The model under review builds one solid part; all positions refer to its coordinate system, in mm. Coordinates: 2 decimals unless noted, no trailing zeros. Order: outer loops, then holes, each group sorted by start corner. A loop starts at its lowest first (then second) coordinate and runs counter-clockwise, first axis right, second up. Notation, with made-up numbers: (69.25, 87.5) - (73.25, 87.5) arc R24 ccw to (73.25, 123.5) - close; hole circle Ø6 at (53, 33.25). An arc over 180 degrees is marked (long way). Answer in a Markdown table with one row per item.
```python
from build123d import *

# Parameters (mm, degrees)
ESQUISSE1_W                  = 70
ESQUISSE1_H                  = 118
BOSS_EXTRU_1_DEPTH           = 3
BOSS_EXTRU_2_DEPTH           = 3
CONG_1_R                     = 3
CONG_2_R                     = 3
CONG_3_R                     = 5
ESQUISSE3_W                  = 70
ESQUISSE3_H                  = 118
BOSS_EXTRU_3_DEPTH           = 3
CONG_4_R                     = 3
ENL_V_MAT_EXTRU_1_DEPTH      = 197.603662224
ENL_V_MAT_EXTRU_1_DEPTH_BACK = 197.603662224


with BuildPart() as part:
    # Esquisse1 → Boss.-Extru.1 (new body)
    with BuildSketch(Plane.XY):
        with Locations((35, 59)):
            Rectangle(ESQUISSE1_W, ESQUISSE1_H)
    extrude(amount=BOSS_EXTRU_1_DEPTH)

    # Esquisse2 → Boss.-Extru.2 (add)
    with BuildSketch(Plane.XY.offset(3)):
        Polygon((0, 118), (7.279404685, 138), (62.720595315, 138), (70, 118), align=None)
        Polygon((0, 118), (-12.5, 113.450372072), (-12.5, 4.549627928), (0, 0), align=None)
        Polygon((65.450372072, -12.5), (4.549627928, -12.5), (0, 0), (70, 0), align=None)
    extrude(amount=-BOSS_EXTRU_2_DEPTH)

    # Congé1
    cong_1_edges = [part.edges().sort_by_distance(p)[0] for p in [
        (-12.5, 4.549627928, 1.5),
        (-12.5, 113.450372072, 1.5),
    ]]
    fillet(cong_1_edges, radius=CONG_1_R)

    # Congé2
    cong_2_edges = [part.edges().sort_by_distance(p)[0] for p in [
        (65.450372072, -12.5, 1.5),
        (4.549627928, -12.5, 1.5),
    ]]
    fillet(cong_2_edges, radius=CONG_2_R)

    # Congé3
    cong_3_edges = [part.edges().sort_by_distance(p)[0] for p in [
        (7.279404685, 138, 1.5),
        (62.720595315, 138, 1.5),
    ]]
    fillet(cong_3_edges, radius=CONG_3_R)

    # Esquisse3 → Boss.-Extru.3 (add)
    with BuildSketch(Plane.XY.offset(3)):
        with Locations((105, 59)):
            Rectangle(ESQUISSE3_W, ESQUISSE3_H)
    extrude(amount=-BOSS_EXTRU_3_DEPTH)

    # Congé4
    cong_4_edges = [part.edges().sort_by_distance(p)[0] for p in [
        (140, 118, 1.5),
        (140, 0, 1.5),
    ]]
    fillet(cong_4_edges, radius=CONG_4_R)

    # Esquisse4 → Enlèv. mat.-Extru.1 (cut, two sides: drawn at the far end of the back side and taken through both)
    with BuildSketch(Plane.XY.offset(3).offset(-ENL_V_MAT_EXTRU_1_DEPTH_BACK)):
        with BuildLine():
            Line((80, 60), (130, 60))
            ThreePointArc((130, 60), (131, 59), (130, 58))
            Line((130, 58), (80, 58))
            ThreePointArc((80, 58), (79, 59), (80, 60))
        make_face()
        with BuildLine():
            Line((80, 40), (130, 40))
            ThreePointArc((130, 40), (131, 39), (130, 38))
            Line((130, 38), (80, 38))
            ThreePointArc((80, 38), (79, 39), (80, 40))
        make_face()
        with BuildLine():
            Line((80, 20), (130, 20))
            ThreePointArc((130, 20), (131, 19), (130, 18))
            Line((130, 18), (80, 18))
            ThreePointArc((80, 18), (79, 19), (80, 20))
        make_face()
    extrude(amount=ENL_V_MAT_EXTRU_1_DEPTH + ENL_V_MAT_EXTRU_1_DEPTH_BACK, mode=Mode.SUBTRACT)


solid = part.part
```
Item 1: We need section B-B, the plane x = 76.5. Write out the cut boundary in (y, z), then the cut area to 3 significant figures.
Check values:
| item | result |
|---|---|
| outline | (0, 0) - (118, 0) - (118, 3) - (0, 3) - close |
| area | 354 mm^2 |
Item 2: We need section A-A, the plane z = 0.6. State how many separate pieces and enclosed holes the cut face has, then the cut area to 3 significant figures.
Check values:
| item | result |
|---|---|
| separate pieces | 1 |
| enclosed holes | 3 |
| area | 19,700 mm^2 |
Item 3: We need section C-C, the plane x = -2. Write out the cut boundary in (y, z).
Check values:
| item | result |
|---|---|
| outline | (0.73, 0) - (117.27, 0) - (117.27, 3) - (0.73, 3) - close |
Item 4: Clearance check with flat-ended pins moving along their axes: pin 1 Ø0.9 at (x, z) = (115, 1) entering from +Y; pin 2 Ø0.9 at (x, z) = (99, 1) entering from -Y. State where each tip first meets the part, or that it passes through.
Check values:
| item | result |
|---|---|
| pin 1 | y = 118 |
| pin 2 | y = 0 |
Item 5: To check wall thickness, follow line 1 (Y direction, x = 109, z = 2.55); line 2 (X direction, y = 112.5, z = 0.9); line 3 (X direction, y = 5, z = 1.5). State the ranges of each line that lie inside material, in increasing order. Write a range as from..to.
Check values:
| item | result |
|---|---|
| line 1 | 0..18, 20..38, 40..58, 60..118 |
| line 2 | -12.27..140 |
| line 3 | -12.01..140 |
